Source: CAD feature listing. Evaluate the final solid. Frame: model axes, mm. A direction names the side the tool comes from. Give positions to 0.01 mm unless a question says otherwise; leave off trailing zeros. Write each loop counter-clockwise with the first axis right and the second up, starting at its lowest first coordinate (ties: lowest second). Pieces come first, ordered by that corner, then holes. Notation, with made-up numbers: (19, 70.25) - (40, 70.25) arc R7 cw to (40, 79.25) - close; hole circle Ø1 at (6, 21.25). An arc over 180 degrees is marked (long way). Answer as a JSON object with one key per item and string values. Group by question number.
from build123d import *

# Parameters (mm, degrees)
BOSS_EXTRUDE1_DEPTH = 18
SKETCH2_R           = 1.7
CUT_EXTRUDE1_DEPTH  = 31.5
CUT_EXTRUDE2_DEPTH  = 1
CUT_EXTRUDE3_DEPTH  = 5


with BuildPart() as part:
    # Sketch1 → Boss-Extrude1 (new body)
    with BuildSketch(Plane(origin=(0, 0, 0), x_dir=(1, 0, 0), z_dir=(0, 1, 0))):
        with BuildLine():
            Line((-16.998275301, 32.528571429), (-32.998275301, 32.528571429))
            Line((-32.998275301, 32.528571429), (-32.998275301, 18.494895774))
            ThreePointArc((-32.998275301, 18.494895774), (-47.498275301, -7.471428571), (-32.998275301, -33.437752917))
            Line((-32.998275301, -33.437752917), (-32.998275301, -47.471428571))
            Line((-32.998275301, -47.471428571), (-16.998275301, -47.471428571))
            Line((-16.998275301, -47.471428571), (-16.998275301, -30.971428571))
            ThreePointArc((-16.998275301, -30.971428571), (-40.498275301, -7.471428571), (-16.998275301, 16.028571429))
            Line((-16.998275301, 16.028571429), (-16.998275301, 32.528571429))
        make_face()
    extrude(amount=BOSS_EXTRUDE1_DEPTH)

    # Sketch2 → Cut-Extrude1 (cut, through all)
    with BuildSketch(Plane(origin=(-16.998275301, 0, 0), x_dir=(0, 0, -1), z_dir=(1, 0, 0))):
        with Locations((-42.471428571, 5.25)):
            Circle(SKETCH2_R)
        with Locations((27.528571429, 5.25)):
            Circle(SKETCH2_R)
    extrude(amount=-CUT_EXTRUDE1_DEPTH, mode=Mode.SUBTRACT)

    # Sketch3 → Cut-Extrude2 (cut)
    with BuildSketch(Plane(origin=(-16.998275301, 0, 0), x_dir=(0, 0, -1), z_dir=(1, 0, 0))):
        Polygon((-41.871148795, 15.201025034), (-39.293157342, 15.201025034), (-39.293157342, 14.251238709), (-40.92136247, 14.251238709), (-40.92136247, 13.233610504), (-39.293157342, 13.233610504), (-39.293157342, 12.283824179), (-40.92136247, 12.283824179), (-40.92136247, 9.909358367), (-41.871148795, 9.909358367), align=None)
        with BuildLine():
            Line((-37.529268453, 13.912029308), (-38.479054777, 13.912029308))
            add(Edge.make_bspline(
                [(-38.479054777, 13.912029308), (-38.472348925, 13.959505738), (-38.459202545, 14.052580134), (-38.427745016, 14.187328674), (-38.390118416, 14.315146885), (-38.34314353, 14.435629995), (-38.288049629, 14.548992623), (-38.225396959, 14.655623774), (-38.154508221, 14.755065768), (-38.100171252, 14.814970019), (-38.073063525, 14.844855162)],
                knots=[0, 0, 0, 0, 0.000143778, 0.000281867, 0.000414671, 0.000543215, 0.000669322, 0.0007924, 0.000913902, 0.001034861, 0.001034861, 0.001034861, 0.001034861], degree=3))
            add(Edge.make_bspline(
                [(-38.073063525, 14.844855162), (-38.033964221, 14.884286443), (-37.956903602, 14.962001353), (-37.82812627, 15.061545568), (-37.693143844, 15.147694317), (-37.549249192, 15.215993668), (-37.398681424, 15.27127408), (-37.240243172, 15.308406058), (-37.074581872, 15.333043453), (-36.961538875, 15.335470322), (-36.903851118, 15.336708795)],
                knots=[0, 0, 0, 0, 0.000166428, 0.000328012, 0.000487119, 0.000645947, 0.000804887, 0.000967376, 0.001133328, 0.001306272, 0.001306272, 0.001306272, 0.001306272], degree=3))
            add(Edge.make_bspline(
                [(-36.903851118, 15.336708795), (-36.852563734, 15.335498), (-36.751743072, 15.333117822), (-36.603562067, 15.314011042), (-36.462283879, 15.280499879), (-36.326415158, 15.236684784), (-36.197954088, 15.177067025), (-36.07406541, 15.107863497), (-35.958210577, 15.022982493), (-35.850118512, 14.927075501), (-35.750815335, 14.8233427), (-35.664818348, 14.712460867), (-35.590885195, 14.597391911), (-35.529974057, 14.477179826), (-35.483141668, 14.3516212), (-35.450638602, 14.221441367), (-35.429364556, 14.08692758), (-35.427245105, 13.99550037), (-35.426170162, 13.949130336)],
                knots=[0, 0, 0, 0, 0.000153836, 0.00030241, 0.000447173, 0.000588968, 0.00072986, 0.000871333, 0.001014032, 0.001159723, 0.001304436, 0.001444171, 0.001580024, 0.001714184, 0.00184768, 0.001981114, 0.002116187, 0.002255197, 0.002255197, 0.002255197, 0.002255197], degree=3))
            add(Edge.make_bspline(
                [(-35.426170162, 13.949130336), (-35.428376009, 13.89170491), (-35.432718642, 13.778651902), (-35.468353097, 13.613190424), (-35.524130708, 13.454979724), (-35.604706892, 13.306233407), (-35.705447645, 13.167356277), (-35.829053175, 13.042991412), (-35.972002875, 12.931188942), (-36.079317119, 12.87110628), (-36.134269788, 12.840339604)],
                knots=[0, 0, 0, 0, 0.00017212, 0.000338852, 0.000505492, 0.00067385, 0.000844528, 0.001018431, 0.001198237, 0.00138694, 0.00138694, 0.00138694, 0.00138694], degree=3))
            add(Edge.make_bspline(
                [(-36.134269788, 12.840339604), (-36.096551119, 12.827955771), (-36.022435626, 12.803622094), (-35.917089364, 12.755697192), (-35.816917106, 12.703323219), (-35.723643783, 12.642478468), (-35.636341679, 12.575623232), (-35.555542998, 12.502186007), (-35.480764986, 12.422326922), (-35.413228364, 12.335606781), (-35.353286974, 12.243412505), (-35.299504756, 12.147873726), (-35.255238993, 12.047541582), (-35.21774038, 11.943561934), (-35.189191072, 11.835000267), (-35.169089807, 11.722277248), (-35.157470783, 11.605650007), (-35.155698684, 11.526635122), (-35.154802641, 11.486682085)],
                knots=[0, 0, 0, 0, 0.000119012, 0.000233852, 0.000346714, 0.000457856, 0.00056747, 0.000676282, 0.000785032, 0.000895296, 0.001005549, 0.001114686, 0.001223822, 0.001334132, 0.001445978, 0.001560132, 0.001677317, 0.001797176, 0.001797176, 0.001797176, 0.001797176], degree=3))
            add(Edge.make_bspline(
                [(-35.154802641, 11.486682085), (-35.156619041, 11.427967343), (-35.160200611, 11.31219383), (-35.182970562, 11.141671293), (-35.225364107, 10.979093204), (-35.281135164, 10.822588857), (-35.355527701, 10.674178666), (-35.443075211, 10.53045682), (-35.55068869, 10.396407552), (-35.670282595, 10.268486948), (-35.803098598, 10.152187262), (-35.947092752, 10.051360668), (-36.09909875, 9.964833512), (-36.260078289, 9.8945883), (-36.429975443, 9.840491454), (-36.608411526, 9.801387759), (-36.796136276, 9.777463472), (-36.924273105, 9.774955464), (-36.989713498, 9.773674607)],
                knots=[0, 0, 0, 0, 0.000176169, 0.00034737, 0.00051474, 0.000679386, 0.000844836, 0.001011921, 0.001183269, 0.001359492, 0.001536793, 0.001711778, 0.001885991, 0.002060677, 0.00223768, 0.002420033, 0.00260805, 0.002804296, 0.002804296, 0.002804296, 0.002804296], degree=3))
            add(Edge.make_bspline(
                [(-36.989713498, 9.773674607), (-37.051619054, 9.775025054), (-37.172667177, 9.777665676), (-37.349725391, 9.800521596), (-37.518002464, 9.837390049), (-37.677927841, 9.889359191), (-37.828882784, 9.956754287), (-37.972236212, 10.037006724), (-38.105127537, 10.134745277), (-38.229037432, 10.245557842), (-38.341217201, 10.369883248), (-38.441479496, 10.504841559), (-38.527613517, 10.650945966), (-38.599972501, 10.80757225), (-38.657990763, 10.974995181), (-38.703755398, 11.152874295), (-38.735722744, 11.341557113), (-38.745458467, 11.471374906), (-38.750422299, 11.537563496)],
                knots=[0, 0, 0, 0, 0.000185653, 0.000363021, 0.000534566, 0.000701839, 0.000866512, 0.001029812, 0.001193709, 0.001360353, 0.001527707, 0.001695195, 0.001863902, 0.002035591, 0.002211932, 0.002394731, 0.002586078, 0.002785121, 0.002785121, 0.002785121, 0.002785121], degree=3))
            Line((-38.750422299, 11.537563496), (-37.800635974, 11.537563496))
            add(Edge.make_bspline(
                [(-37.800635974, 11.537563496), (-37.794617277, 11.504283004), (-37.782894287, 11.439460519), (-37.760029312, 11.345611971), (-37.730233061, 11.258983964), (-37.695781181, 11.178806552), (-37.658567964, 11.104027033), (-37.613605499, 11.037407199), (-37.564188399, 10.977138049), (-37.492879164, 10.905489419), (-37.3909377, 10.831873443), (-37.253282951, 10.767897658), (-37.100155079, 10.730399988), (-36.993103425, 10.725825387), (-36.937772058, 10.723460932)],
                knots=[0, 0, 0, 0, 0.000101453, 0.000197607, 0.000289457, 0.000375893, 0.000459333, 0.000539595, 0.000616416, 0.00069287, 0.00084235, 0.000990791, 0.001145821, 0.001311674, 0.001311674, 0.001311674, 0.001311674], degree=3))
            add(Edge.make_bspline(
                [(-36.937772058, 10.723460932), (-36.90841128, 10.72396442), (-36.850900082, 10.724950642), (-36.766424697, 10.735881586), (-36.685949998, 10.753884861), (-36.609326097, 10.778350644), (-36.536065202, 10.809020032), (-36.467567036, 10.848566373), (-36.402435434, 10.89454464), (-36.341378437, 10.946236417), (-36.284960514, 11.002561951), (-36.238017483, 11.06493291), (-36.19511495, 11.128312952), (-36.163383928, 11.196848623), (-36.135580716, 11.266851971), (-36.11856373, 11.340863899), (-36.105714684, 11.417331835), (-36.104967949, 11.469663134), (-36.104588966, 11.49622235)],
                knots=[0, 0, 0, 0, 8.804e-05, 0.00017245, 0.000255004, 0.000335125, 0.000413489, 0.000492771, 0.000571884, 0.000652369, 0.000732575, 0.000810392, 0.000886249, 0.00096163, 0.001036443, 0.001111772, 0.00118898, 0.001268546, 0.001268546, 0.001268546, 0.001268546], degree=3))
            add(Edge.make_bspline(
                [(-36.104588966, 11.49622235), (-36.105595096, 11.525269377), (-36.10759807, 11.583095353), (-36.123962582, 11.667480206), (-36.149805605, 11.748651634), (-36.18570472, 11.82625017), (-36.233643988, 11.899989803), (-36.290211789, 11.971349973), (-36.35986473, 12.036616511), (-36.436283336, 12.101130505), (-36.524898897, 12.15736725), (-36.621395711, 12.209265504), (-36.728309865, 12.250560491), (-36.843031489, 12.287444563), (-36.967730649, 12.314384117), (-37.101633011, 12.333944858), (-37.244522568, 12.348504799), (-37.343018198, 12.350593662), (-37.393584692, 12.35166606)],
                knots=[0, 0, 0, 0, 8.7084e-05, 0.000173364, 0.000256838, 0.000342201, 0.000428949, 0.000520167, 0.000614623, 0.000714788, 0.000819753, 0.000928812, 0.001042981, 0.001163003, 0.001290052, 0.001425126, 0.001568892, 0.001720568, 0.001720568, 0.001720568, 0.001720568], degree=3))
            Line((-37.393584692, 12.35166606), (-37.393584692, 13.233610504))
            add(Edge.make_bspline(
                [(-37.393584692, 13.233610504), (-37.330626399, 13.238972234), (-37.212843901, 13.249002968), (-37.049355478, 13.272460189), (-36.911719301, 13.303814627), (-36.796627281, 13.34164206), (-36.701062242, 13.390222338), (-36.617577152, 13.44385282), (-36.545675843, 13.506136787), (-36.484909592, 13.57521694), (-36.436298482, 13.649402546), (-36.40189437, 13.727540541), (-36.379175692, 13.80721324), (-36.377023099, 13.861706965), (-36.375956487, 13.888708661)],
                knots=[0, 0, 0, 0, 0.000189544, 0.000354599, 0.000494992, 0.000612655, 0.000716948, 0.000815736, 0.000909673, 0.001001315, 0.001090992, 0.001174513, 0.001256793, 0.001337606, 0.001337606, 0.001337606, 0.001337606], degree=3))
            add(Edge.make_bspline(
                [(-36.375956487, 13.888708661), (-36.377796698, 13.923159894), (-36.3813884, 13.990401408), (-36.409283508, 14.086638178), (-36.457706253, 14.172425283), (-36.522632653, 14.247582201), (-36.601747728, 14.310358892), (-36.694484465, 14.355933699), (-36.798830471, 14.382710933), (-36.872243509, 14.38548683), (-36.910211295, 14.38692247)],
                knots=[0, 0, 0, 0, 0.000103264, 0.00020155, 0.000297405, 0.00039663, 0.000497784, 0.000598286, 0.000704469, 0.000818208, 0.000818208, 0.000818208, 0.000818208], degree=3))
            add(Edge.make_bspline(
                [(-36.910211295, 14.38692247), (-36.944624824, 14.385228566), (-37.012911806, 14.381867343), (-37.112767812, 14.356780059), (-37.20759775, 14.314548739), (-37.295437959, 14.256314238), (-37.375020447, 14.18637707), (-37.440334709, 14.103551012), (-37.494660015, 14.012798316), (-37.517687082, 13.945750658), (-37.529268453, 13.912029308)],
                knots=[0, 0, 0, 0, 0.000103172, 0.000204725, 0.000306758, 0.000413189, 0.000519795, 0.000623097, 0.000728547, 0.000835248, 0.000835248, 0.000835248, 0.000835248], degree=3))
        make_face()
    extrude(amount=-CUT_EXTRUDE2_DEPTH, mode=Mode.SUBTRACT)

    # Sketch4 → Cut-Extrude3 (cut)
    with BuildSketch(Plane.ZY.offset(32.998275301)):
        Polygon((-25.528765418, 2.783401278), (-24.392531269, 5.748583447), (-26.39233728, 8.215182169), (-29.528377439, 7.716598722), (-30.664611588, 4.751416553), (-28.664805577, 2.284817831), align=None)
        Polygon((44.362800811, 2.699305117), (45.626081257, 5.612628966), (43.734709018, 8.163323849), (40.580056332, 7.800694883), (39.316775886, 4.887371034), (41.208148125, 2.336676151), align=None)
    extrude(amount=-CUT_EXTRUDE3_DEPTH, mode=Mode.SUBTRACT)


solid = part.part
Q1. Section D-D on z = -10. Return the cut outline in (x, y).
Q2. Reachability of faces 1 (the flat face through (-32.998, 9, -26)), 2 (the flat face through (-30.53, 6.25, -30.09)), 3 (the cylindrical face through (-22.42, 3.74, -28.31)), 4 (the flat face through (-32.998, 9, 40)), 5 (the flat face through (-16.998, 9, 39)) from +Z, -Z, +X, -X, +Y, -Y: full face, straight path, thin tool, end or side. Return the list, or none.
Q3. Draft query along Y for faces 6 (the flat face through (-43, 0, 7)), 7 (the flat face through (-30.53, 7.97, -27.94)), 8 (the cylindrical face through (-40.493, 8.874, 7.988)). Return one class per face: released by +Y, released by -Y, zero draft, split by the parting line, or undercut.
Q4. Section B-B on x = -24. Return the cut outline in (y, z), then the cut area to 3 significant figures.
Q5. Ray query, probe 1 along Z at (x, y) = (-26.5, 4); probe 2 along Z at (x, y) = (-28, 14); probe 3 along X at (y, z) = (12.75, -27). Return the intervals inside material, ascending. Write a range as [from, to].
Q6. First-contact query: pin 1 Ø1 at (y, z) = (10, 3.5) entering from -X; pin 2 Ø5 at (y, z) = (15.5, -24) entering from -X; pin 3 Ø6 at (y, z) = (12.5, 27.5) entering from -X. Flat tips, straight axial feed; report the tip coordinate or a pass-through.
Q7. Section A-A on x = -34.5. Return the cut outline in (y, z), then the cut area to 3 significant figures.
Q8. Section C-C on z = -20. Return the cut outline in (x, y), then the cut area to 3 significant figures.
Taken from the geometry:
{
 "1": {"outline": "(-42, 0) - (-32.71, 0) - (-32.71, 18) - (-42, 18) - close"},
 "2": {"face 1": "-Z, -X, +Y, -Y", "face 2": "-X", "face 3": "+X, -X", "face 4": "+Z, -X, +Y, -Y", "face 5": "+Z, -Z, +X, +Y, -Y"},
 "3": {"face 6": "released by -Y", "face 7": "undercut", "face 8": "zero draft"},
 "4": {"outline": "(0, -32.53) - (18, -32.53) - (18, -14.96) - (0, -14.96) - close; (0, 29.9) - (18, 29.9) - (18, 47.47) - (0, 47.47) - close; hole circle Ø3.4 at (5.25, -27.53); hole circle Ø3.4 at (5.25, 42.47)", "area": "614 mm²"},
 "5": {"probe 1": "z = [-32.53, -28.68], [-26.38, -14.02], [28.96, 41.32], [43.62, 47.47]", "probe 2": "z = [-32.53, -13.29], [28.24, 47.47]", "probe 3": "x = [-33, -17]"},
 "6": {"pin 1": "stops at x = -47.3", "pin 2": "stops at x = -33", "pin 3": "stops at x = -42.3"},
 "7": {"outline": "(0, -17.51) - (18, -17.51) - (18, -8.21) - (0, -8.21) - close; (0, 23.15) - (18, 23.15) - (18, 32.45) - (0, 32.45) - close", "area": "335 mm²"},
 "8": {"outline": "(-33, 0) - (-17, 0) - (-17, 18) - (-33, 18) - close", "area": "288 mm²"}
}
